```python
from build123d import *

# Parameters (mm, degrees)
F1_DEPTH = 1.6
F3_DEPTH = 1.601


with BuildPart() as f1:
    # F0 (on Top) → F1 (new body)
    with BuildSketch(Plane.XY):
        Polygon((17.4, -14.125), (-17.4, 14.125), (-17.4, -14.125), align=None)
        Polygon((17.4, 14.125), (-17.4, 14.125), (17.4, -14.125), align=None)
    extrude(amount=F1_DEPTH)

    # F2 (on face) → F3 (cut, through all)
    with BuildSketch(Plane.XY.offset(1.6)):
        with BuildLine():
            ThreePointArc((-12.3, 10.125), (-14.177817, 10.902817), (-13.4, 9.025))
            Line((-13.4, 9.025), (-13.4, 10.125))
            Line((-13.4, 10.125), (-12.3, 10.125))
        make_face()
        with BuildLine():
            Line((-13.4, 10.125), (-13.4, 9.025))
            ThreePointArc((-13.4, 9.025), (-12.622183, 9.347183), (-12.3, 10.125))
            Line((-12.3, 10.125), (-13.4, 10.125))
        make_face()
        with BuildLine():
            ThreePointArc((-13.4, -9.025), (-14.177817, -10.902817), (-12.3, -10.125))
            Line((-12.3, -10.125), (-13.4, -10.125))
            Line((-13.4, -10.125), (-13.4, -9.025))
        make_face()
        with BuildLine():
            Line((-13.4, -10.125), (-12.3, -10.125))
            ThreePointArc((-12.3, -10.125), (-12.622183, -9.347183), (-13.4, -9.025))
            Line((-13.4, -9.025), (-13.4, -10.125))
        make_face()
        with BuildLine():
            Line((13.4, -10.125), (12.3, -10.125))
            ThreePointArc((12.3, -10.125), (13.4, -11.225), (14.5, -10.125))
            ThreePointArc((14.5, -10.125), (14.177817, -9.347183), (13.4, -9.025))
            Line((13.4, -9.025), (13.4, -10.125))
        make_face()
        with BuildLine():
            ThreePointArc((13.4, -9.025), (12.622183, -9.347183), (12.3, -10.125))
            Line((12.3, -10.125), (13.4, -10.125))
            Line((13.4, -10.125), (13.4, -9.025))
        make_face()
        with BuildLine():
            Line((13.4, 10.125), (13.4, 9.025))
            ThreePointArc((13.4, 9.025), (14.177817, 9.347183), (14.5, 10.125))
            ThreePointArc((14.5, 10.125), (13.4, 11.225), (12.3, 10.125))
            Line((12.3, 10.125), (13.4, 10.125))
        make_face()
        with BuildLine():
            ThreePointArc((12.3, 10.125), (12.622183, 9.347183), (13.4, 9.025))
            Line((13.4, 9.025), (13.4, 10.125))
            Line((13.4, 10.125), (12.3, 10.125))
        make_face()
    extrude(amount=-F3_DEPTH, mode=Mode.SUBTRACT)


solid = f1.part
```
Can you work these out from the model? Positions are in its coordinate system, mm. Give positions to 0.01 mm unless a question says otherwise; leave off trailing zeros. Write each loop counter-clockwise with the first axis right and the second up, starting at its lowest first coordinate (ties: lowest second). Pieces come first, ordered by that corner, then holes. Notation, with made-up numbers: (52, 74) -> (84, 74) arc R22 ccw to (84, 82) -> close; hole circle Ø9 at (32, -18). An arc over 180 degrees is marked (long way). Write item = value, one per line.
(1) Suppose I cut it at B-B on x = 14. Write out the boundary of the cut face in (y, z) (3 decimals).
Worked out:
outline = (-14.125, 0) -> (-11.047, 0) -> (-11.047, 1.6) -> (-14.125, 1.6) -> close; (-9.203, 0) -> (9.203, 0) -> (9.203, 1.6) -> (-9.203, 1.6) -> close; (11.047, 0) -> (14.125, 0) -> (14.125, 1.6) -> (11.047, 1.6) -> close
(2) Suppose I cut it at A-A on z = 0.65. Write out the boundary of the cut face in (x, y) (3 decimals), then the cut area to 3 significant figures.
Worked out:
outline = (-17.4, -14.125) -> (17.4, -14.125) -> (17.4, 14.125) -> (-17.4, 14.125) -> close; hole (-13.4, -9.025) arc R1.1 ccw (long way) to (-12.3, -10.125) arc R1.1 ccw to start; hole (-13.4, 9.025) arc R1.1 ccw to (-12.3, 10.125) arc R1.1 ccw (long way) to start; hole (12.3, -10.125) arc R1.1 ccw to (14.5, -10.125) arc R1.1 ccw to (13.4, -9.025) arc R1.1 ccw to start; hole (12.3, 10.125) arc R1.1 ccw to (13.4, 9.025) arc R1.1 ccw to (14.5, 10.125) arc R1.1 ccw to start
area = 968 mm^2
(3) Suppose I cut it at C-C on y = -10.75. Write out the boundary of the cut face in (x, z).
Worked out:
outline = (-17.4, 0) -> (-14.31, 0) -> (-14.31, 1.6) -> (-17.4, 1.6) -> close; (-12.49, 0) -> (12.49, 0) -> (12.49, 1.6) -> (-12.49, 1.6) -> close; (14.31, 0) -> (17.4, 0) -> (17.4, 1.6) -> (14.31, 1.6) -> close
(4) I need wall thicknesses on probe 1 along Y at (x, z) = (-13.4, 1) (3 decimals); probe 2 along X at (y, z) = (9.25, 0.6). Which ranges of each line are inside material? Lowest first, please. Write a range as from..to.
Worked out:
probe_1 = -14.125..-11.225, -9.025..9.025, 11.225..14.125
probe_2 = -17.4..-14.07, -12.73..12.73, 14.07..17.4
(5) I'm going to push a flat-ended pin straight in: P1, Ø10, axis at x = 12, y = -5, coming from the -Z side. Where does the tip first touch, or does it pass through?
Worked out:
P1 = 0
